from build123d import *

# Parameters (mm, degrees)
BOSS_EXTRUDE1_DEPTH            = 11
CBORE_FOR_M4_SHCS2_D           = 4.5
CBORE_FOR_M4_SHCS2_CBORE_D     = 8
CBORE_FOR_M4_SHCS2_CBORE_DEPTH = 11.079
FILLET1_R                      = 0.5


with BuildPart() as part:
    # Sketch1 → Boss-Extrude1 (new body)
    with BuildSketch(Plane.XY):
        with BuildLine():
            ThreePointArc((0.381, 5.987891031), (3.163547137, 5.098231998), (5.196152423, 3))
            ThreePointArc((5.196152423, 3), (5.795554958, 1.552914271), (6, 0))
            ThreePointArc((6, 0), (5.795554958, -1.552914271), (5.196152423, -3))
            ThreePointArc((5.196152423, -3), (3.163547137, -5.098231998), (0.381, -5.987891031))
            Line((0.381, -5.987891031), (0.381, -7.765891031))
            Line((0.381, -7.765891031), (-0.381, -7.765891031))
            Line((-0.381, -7.765891031), (-0.381, -5.987891031))
            ThreePointArc((-0.381, -5.987891031), (-6, 0), (-0.381, 5.987891031))
            Line((-0.381, 5.987891031), (-0.381, 13.994814718))
            ThreePointArc((-0.381, 13.994814718), (-9.763861941, -10.033294574), (14, 0))
            ThreePointArc((14, 0), (10.033294574, 9.763861941), (0.381, 13.994814718))
            Line((0.381, 13.994814718), (0.381, 5.987891031))
        make_face()
    extrude(amount=BOSS_EXTRUDE1_DEPTH)

    # CBORE for M4 SHCS2 (through all)
    with Locations(Plane(origin=(14, 0, 0), x_dir=(0, 0, 1), z_dir=(1, 0, 0))):
        with Locations((5.5, -9.991352875)):
            CounterBoreHole(CBORE_FOR_M4_SHCS2_D / 2, CBORE_FOR_M4_SHCS2_CBORE_D / 2, CBORE_FOR_M4_SHCS2_CBORE_DEPTH)

    # Fillet1
    fillet1_edges = [part.edges().sort_by_distance(p)[0] for p in [
        (-9.763861941, -10.033294574, 11),
        (-9.763861941, -10.033294574, 0),
    ]]
    fillet(fillet1_edges, radius=FILLET1_R)


solid = part.part
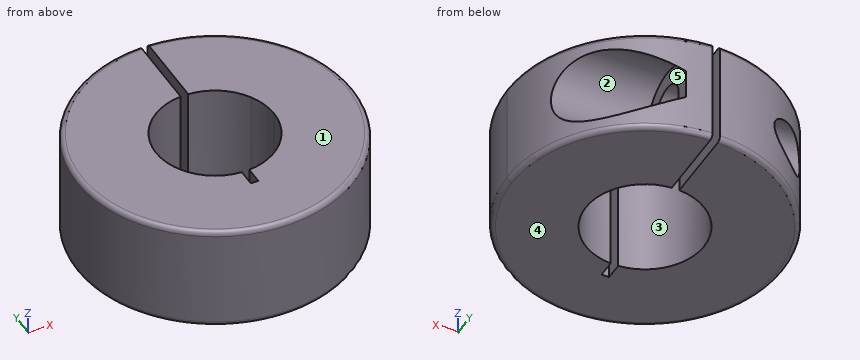
Read the model definition and answer for the solid it produces. Units are mm, in the model's axes. Face numbers are marked on the shaded views. A direction names the side the tool comes from. Give positions to 0.01 mm unless a question says otherwise; leave off trailing zeros. Write each loop counter-clockwise with the first axis right and the second up, starting at its lowest first coordinate (ties: lowest second). Pieces come first, ordered by that corner, then holes. Notation, with made-up numbers: (61.5, 38.25) - (108.5, 38.25) arc R23 ccw to (108.5, 69.25) - close; hole circle Ø6 at (24.5, -9). An arc over 180 degrees is marked (long way). Use CSV: the item, a comma, the result in double quotes. Start each with the question number.
Item 1: Consider line 1 (Y direction, x = 0.5, z = 3.75); line 2 (X direction, y = 12.75, z = 3); line 3 (Y direction, x = 1.5, z = 3). Determine where each line is inside the solid, lowest interval first.
Item 2: For the marked faces 1, 2 and 3, determine the directions among +Z, -Z, +X, -X, +Y, -Y from which every point of the face is accessible in a straight line to the end or side of a thin tool.
Item 3: The part is cut by section D-D, the plane z = 2. Give the vertices of the cut face in (x, y), and give its area (3 significant figures).
Item 4: Flat-ended cylindrical pins translate along their axes: P1, Ø0.5, axis at y = -7, z = 6.5, coming from the +X side; P2, Ø5, axis at x = 4, z = 7.5, coming from the +Y side; P3, Ø4, axis at y = 11.5, z = 6.5, coming from the +X side. Find the tip coordinate at first contact, or state that the pin passes through.
Item 5: The part is cut by section A-A, the plane z = 5.5. Give the vertices of the cut face in (x, y).
Item 6: The mould has two halves that part along Y. Classify the marked faces 4 and 5: pulls with the +Y half, pulls with the -Y half, needs draft (parallel to the pull), parting line crosses it, or undercut.
Item 7: The part is cut by section B-B, the plane x = 1.25. Count the separate pieces of the cut face and the enclosed holes in it, and give its area (3 significant figures).
Taken from the geometry:
1,line 1,"-13.99 to -5.98, 5.98 to 8.58, 11.41 to 13.99"
1,line 2,"-5.78 to -0.38, 0.38 to 2.92"
1,line 3,"-13.92 to -5.81, 5.81 to 13.92"
2,face 1,"+Z, +X, -X, +Y, -Y"
2,face 2,"+X"
2,face 3,"+Z, -Z"
3,outline,"(-0.38, -7.77) - (-0.38, -5.99) arc R6 cw to (-0.38, 5.99) - (-0.38, 13.99) arc R14 ccw (long way) to (11.45, 8.05) - (2.92, 8.05) - (2.92, 11.93) - (7.33, 11.93) arc R14 ccw to (0.38, 13.99) - (0.38, 5.99) arc R6 cw to (0.38, -5.99) - (0.38, -7.77) - close"
3,area,"469 mm2"
4,P1,"x = 12.27"
4,P2,"y = 13.92"
4,P3,"x = 2.92"
5,outline,"(-11.66, 7.74) arc R14 ccw (long way) to (12.65, 5.99) - (2.92, 5.99) - (2.92, 7.74) - (0.38, 7.74) - (0.38, 5.99) arc R6 cw to (0.38, -5.99) - (0.38, -7.77) - (-0.38, -7.77) - (-0.38, -5.99) arc R6 cw to (-0.38, 5.99) - (-0.38, 7.74) - close; (-6.79, 12.24) - (-0.38, 12.24) - (-0.38, 13.99) arc R14 ccw to start; (0.38, 12.24) - (2.92, 12.24) - (2.92, 13.69) arc R14 ccw to (0.38, 13.99) - close"
6,face 4,"needs draft"
6,face 5,"undercut"
7,separate pieces,"2"
7,enclosed holes,"1"
7,area,"162 mm2"
